Can you work these out from the model? Positions are in its coordinate system, mm. A direction names the side the tool comes from. Coordinates: 2 decimals unless noted, no trailing zeros. Loops run counter-clockwise (first coordinate to the right, second up) from the corner with the lowest first, then second, coordinate; pieces in that order, holes last. Notation, with made-up numbers: (7.5, 77) - (66.5, 77) arc R14 ccw to (66.5, 89) - close; hole circle Ø8 at (17, 85). An arc over 180 degrees is marked (long way). Put each result on its own line as item: value. Start each with the question number.
from build123d import *

# Parameters (mm, degrees)
F1_DEPTH = 6
F2_R     = 1.75
F3_DEPTH = 6.001
F4_W     = 10
F4_H     = 10
F5_DEPTH = 6.001


with BuildPart() as f1:
    # F0 (on Front) → F1 (new body)
    with BuildSketch(Plane.XZ):
        with BuildLine():
            Line((-68, 0), (0, 0))
            Line((0, 0), (68, 0))
            Line((68, 0), (68, 62))
            Line((68, 62), (47.25, 62))
            Line((47.25, 62), (47.25, 53.147458))
            Line((47.25, 53.147458), (34.951913, 31.964558))
            ThreePointArc((34.951913, 31.964558), (31.486373, 27.742888), (26.860942, 24.838089))
            Line((26.860942, 24.838089), (0, 13.5))
            Line((0, 13.5), (-26.860942, 24.838089))
            ThreePointArc((-26.860942, 24.838089), (-31.486373, 27.742888), (-34.951913, 31.964558))
            Line((-34.951913, 31.964558), (-47.25, 53.147458))
            Line((-47.25, 53.147458), (-47.25, 62))
            Line((-47.25, 62), (-68, 62))
            Line((-68, 62), (-68, 0))
        make_face()
    extrude(amount=F1_DEPTH)

    # F2 (on face) → F3 (cut, through all)
    with BuildSketch(Plane.XZ.offset(6)):
        with Locations((-51.5, 54.25)):
            Circle(F2_R)
        with Locations((-51.5, 16.75)):
            Circle(F2_R)
        with Locations((51.5, 54.25)):
            Circle(F2_R)
        with Locations((51.5, 16.75)):
            Circle(F2_R)
    extrude(amount=-F3_DEPTH, mode=Mode.SUBTRACT)

    # F4 (on face) → F5 (cut, through all)
    with BuildSketch(Plane.XZ.offset(6)):
        with Locations((-47.25, 5)):
            Rectangle(F4_W, F4_H)
        with Locations((47.25, 5)):
            Rectangle(F4_W, F4_H)
    extrude(amount=-F5_DEPTH, mode=Mode.SUBTRACT)


solid = f1.part
Q1. I want a section at C-C on y = -2. List the corners of the cut face in (x, z) for me, and give its area (3 significant figures).
Q2. I want a section at A-A on z = 4. List the corners of the cut face in (x, y) for me.
Q3. We'd pull the mould along X, two halves only. Please class faces 1 (the flat face through (68, -3, 31)), 2 (the flat face through (-52.25, -3, 5)), 3 (the flat face through (-1, 0, 11)): released by +X, released by -X, zero draft, split by the parting line, or undercut.
Q4. Will these pins go through, and if not, where does the flat tip stop? pin 1 (1.5 mm diameter, centred on x = -24.5, y = -4.5, fed in from +Z); pin 2 (3 mm diameter, centred on x = -51.5, z = 16.75, fed in from +Y); pin 3 (1.8 mm diameter, centred on x = -47.5, y = -1.5, fed in from -Z).
Q5. I want a section at D-D on z = 50. List the corners of the cut face in (x, y) for me.
Q6. I want a section at B-B on z = 16.75. List the corners of the cut face in (x, y) for me, and give its area (3 significant figures).
Q7. Please list where these lines run through material, in increasing order: line 1 along X through (y, z) = (-1, 9); line 2 along Z through (x, y) = (51.5, -3.6); line 3 along X through (y, z) = (-4.8, 58). Write a range as [from, to].
Q8. On a 3-axis mill with a long thin cutter (end or side, diameter ignored), from which of +Z, -Z, +X, -X, +Y, -Y can I reach the whole of each face in a straight line? I mean faces 4 (the flat face through (-41.015, -2.958, 42.408)), 5 (the flat face through (-47, -3, 10)), 6 (the cylindrical face through (53.169, -3.042, 17.276)). Say none if no direction works.
Calculated:
1. outline: (-68, 0) - (-52.25, 0) - (-52.25, 10) - (-42.25, 10) - (-42.25, 0) - (42.25, 0) - (42.25, 10) - (52.25, 10) - (52.25, 0) - (68, 0) - (68, 62) - (47.25, 62) - (47.25, 53.15) - (34.95, 31.96) arc R17 cw to (26.86, 24.84) - (0, 13.5) - (-26.86, 24.84) arc R17 cw to (-34.95, 31.96) - (-47.25, 53.15) - (-47.25, 62) - (-68, 62) - close; hole circle Ø3.5 at (-51.5, 16.75); hole circle Ø3.5 at (-51.5, 54.25); hole circle Ø3.5 at (51.5, 16.75); hole circle Ø3.5 at (51.5, 54.25)
1. area: 4,860 mm2
2. outline: (-68, -6) - (-52.25, -6) - (-52.25, 0) - (-68, 0) - close; (-42.25, -6) - (42.25, -6) - (42.25, 0) - (-42.25, 0) - close; (52.25, -6) - (68, -6) - (68, 0) - (52.25, 0) - close
3. face 1: released by +X
3. face 2: undercut
3. face 3: zero draft
4. pin 1: z = 24.16
4. pin 2: through
4. pin 3: z = 10
5. outline: (-68, -6) - (-45.42, -6) - (-45.42, 0) - (-68, 0) - close; (45.42, -6) - (68, -6) - (68, 0) - (45.42, 0) - close
6. outline: (-68, -6) - (-53.25, -6) - (-53.25, 0) - (-68, 0) - close; (-49.75, -6) - (-7.7, -6) - (-7.7, 0) - (-49.75, 0) - close; (7.7, -6) - (49.75, -6) - (49.75, 0) - (7.7, 0) - close; (53.25, -6) - (68, -6) - (68, 0) - (53.25, 0) - close
6. area: 682 mm2
7. line 1: [-68, -52.25], [-42.25, 42.25], [52.25, 68]
7. line 2: [10, 15], [18.5, 52.5], [56, 62]
7. line 3: [-68, -47.25], [47.25, 68]
8. face 4: +Z, +Y, -Y
8. face 5: -Z, +Y, -Y
8. face 6: +Y, -Y
